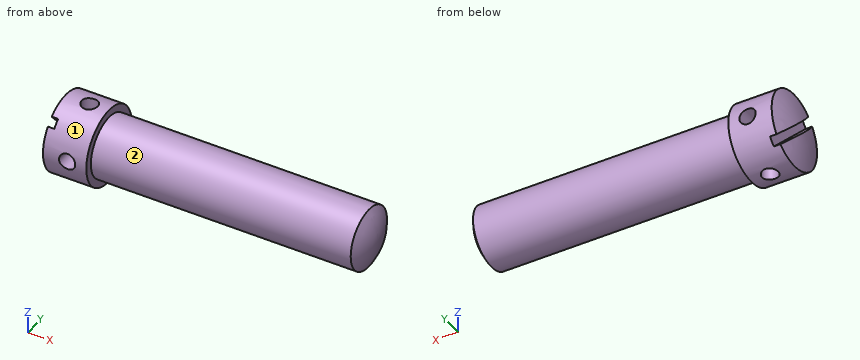
```python
from build123d import *

# Parameters (mm, degrees)
SKETCH2_R          = 4
NECK_DEPTH         = 35
SKETCH5_R          = 1.06
CUT_EXTRUDE1_DEPTH = 70
SKETCH6_R          = 1.06
CUT_EXTRUDE2_DEPTH = 70
SKETCH7_W          = 1.7
SKETCH7_H          = 1.2
CUT_EXTRUDE3_DEPTH = 70
SCALE_1_SCALE      = 1.5


with BuildPart() as part:
    # Sketch1 → BaseHead (revolve)
    with BuildSketch(Plane.XY):
        with BuildLine():
            Line((0.857864376, 5), (6.5, 5))
            Line((6.5, 5), (6.5, 0))
            Line((6.5, 0), (0, 0))
            ThreePointArc((0, 0), (0.216021605, 2.536529681), (0.857864376, 5))
        make_face()
    revolve(axis=Axis((-25.059543495, 0, 0), (1, 0, 0)))

    # Sketch2 → Neck (add)
    with BuildSketch(Plane(origin=(6.5, 3.614329884, 0.195577912), x_dir=(0, 0, -1), z_dir=(1, 0, 0))):
        with Locations(Location((0.195577912, -3.614329884, 0), (0, 0, 180))):
            Circle(SKETCH2_R)
    extrude(amount=NECK_DEPTH)

    # Sketch4 → Cut-Revolve1 (revolve, cut)
    with BuildSketch(Plane.XY, mode=Mode.PRIVATE) as cut_revolve1_sk:
        with BuildLine():
            Line((34, 7.5), (34, 12.5))
            Line((34, 12.5), (46.5, 12.5))
            Line((46.5, 12.5), (46.5, 0))
            Line((46.5, 0), (41.5, 0))
            ThreePointArc((41.5, 0), (39.303300859, 5.303300859), (34, 7.5))
        make_face()
    revolve(cut_revolve1_sk.sketch.rotate(Axis((61.414233577, 0, 0), (-1, 0, 0)), 270), axis=Axis((61.414233577, 0, 0), (-1, 0, 0)), mode=Mode.SUBTRACT)

    # Sketch5 → Cut-Extrude1 (cut, symmetric)
    with BuildSketch(Plane.XY):
        with Locations((4, 0)):
            Circle(SKETCH5_R)
    extrude(amount=CUT_EXTRUDE1_DEPTH, both=True, mode=Mode.SUBTRACT)

    # Sketch6 → Cut-Extrude2 (cut, symmetric)
    with BuildSketch(Plane(origin=(0, 0, 0), x_dir=(1, 0, 0), z_dir=(0, 1, 0))):
        with Locations(Location((4, 0, 0), (0, 0, 270))):
            Circle(SKETCH6_R)
    extrude(amount=CUT_EXTRUDE2_DEPTH, both=True, mode=Mode.SUBTRACT)

    # Sketch7 → Cut-Extrude3 (cut, symmetric)
    with BuildSketch(Plane(origin=(0, 0, 0), x_dir=(1, 0, 0), z_dir=(0, -0.7071067811865488, 0.7071067811865462))):
        with Locations((0.85, 0)):
            Rectangle(SKETCH7_W, SKETCH7_H)
    extrude(amount=CUT_EXTRUDE3_DEPTH, both=True, mode=Mode.SUBTRACT)


with BuildPart() as part_1:
    # 缩放比例1: scaled about (19.948892128, -3.087e-06, -4.178e-06)
    add(part.part.scale(SCALE_1_SCALE).moved(Location((-9.974446064, 1.543e-06, 2.089e-06))))


solid = part_1.part
```
CAD build for the part. Positions are in the model's coordinates, mm. Face numbers are marked on the shaded views. A direction names the side the tool comes from. Round coordinates to 2 decimals unless told otherwise and drop trailing zeros. Order: outer loops, then holes, each group sorted by start corner. A loop starts at its lowest first (then second) coordinate and runs counter-clockwise, first axis right, second up. Notation, with made-up numbers: (-9.5, 66.25) - (38.5, 66.25) arc R25 cw to (38.5, 87.25) - close; hole circle Ø10 at (-22, 22.5). An arc over 180 degrees is marked (long way). Use CSV: the item, a comma, the result in double quotes. Start each with the question number.
1) Saw through at A-A (y = 4). List the corners of the cut face in (x, z).
2) Saw through at C-C (y = -1). List the corners of the cut face in (x, z).
3) Wall check: L1, parallel to X at y = -0.5, z = 2.75; L2, parallel to X at y = -5.5, z = 5; L3, parallel to X at y = 1, z = -1. Give the ranges that are in metal, low to high. Write a range as [from, to].
4) Pin check, flat tips, straight feed: pin 1 Ø5 at (x, y) = (45.5, -5) entering from +Z; pin 2 Ø5 at (x, y) = (30.5, 5.5) entering from +Z; pin 3 Ø6 at (x, y) = (37, -1) entering from -Z. Stop position of each tip, or through.
5) Tool access for the marked faces 1 and 2: list every direction of +Z, -Z, +X, -X, +Y, -Y with a clear straight run to the whole face (end or side of a thin tool).
6) Saw through at B-B (z = -5.25). List the corners of the cut face in (x, y), and give its area (3 significant figures).
Values follow:
1,outline,"(-9.45, -2.73) - (-7.42, -2.73) - (-7.42, -5.27) - (-8.98, -5.27) arc R22.14 ccw to (-8.69, -6.34) - (-0.22, -6.34) - (-0.22, -4.47) - (50.54, -4.47) arc R10.51 ccw to (50.54, 4.47) - (-0.22, 4.47) - (-0.22, 6.34) - (-8.69, 6.34) arc R22.14 ccw to start; hole circle Ø3.18 at (-3.97, 0)"
2,outline,"(-9.95, -0.27) arc R22.48 ccw to (-8.69, -7.43) - (-5.21, -7.43) - (-5.21, -1) arc R1.59 cw to (-5.21, 1) - (-5.21, 7.43) - (-8.69, 7.43) arc R22.48 ccw to (-9.84, 2.27) - (-7.42, 2.27) - (-7.42, -0.27) - close; (-2.74, -7.43) - (-0.22, -7.43) - (-0.22, -5.92) - (50.54, -5.92) arc R11.21 ccw to (50.54, 5.92) - (-0.22, 5.92) - (-0.22, 7.43) - (-2.74, 7.43) - (-2.74, 1) arc R1.59 cw to (-2.74, -1) - close"
3,L1,"x = [-9.8, -5.48], [-2.47, 51.92]"
3,L2,"x = [-7.42, -0.22]"
3,L3,"x = [-7.42, -5.21], [-2.74, 52.19]"
4,pin 1,"stops at z = 5.45"
4,pin 2,"stops at z = 5.2"
4,pin 3,"stops at z = -6"
5,face 1,"+X, -X"
5,face 2,"+X"
6,outline,"(-8.99, 3.98) arc R21.88 ccw to (-8.69, -5.36) - (-0.22, -5.36) - (-0.22, -2.9) - (50.54, -2.9) arc R9.95 ccw to (50.54, 2.9) - (-0.22, 2.9) - (-0.22, 5.36) - (-7.42, 5.36) - (-7.42, 3.98) - close; hole circle Ø3.18 at (-3.97, 0)"
6,area,"382 mm2"
